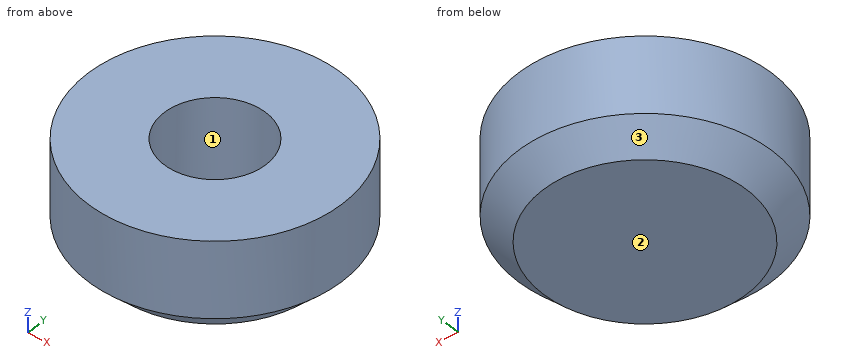
```python
from build123d import *

# Parameters (mm, degrees)
SKETCH_1_R      = 15
EXTRUDE_1_DEPTH = 2
SKETCH_2_R      = 15
SKETCH_2_R_2    = 6
EXTRUDE_2_DEPTH = 10
CHAMFER_1_SIZE  = 3


with BuildPart() as part:
    # 草图1 → 凸台-拉伸1 (new body)
    with BuildSketch(Plane.XY):
        Circle(SKETCH_1_R)
    extrude(amount=EXTRUDE_1_DEPTH)

    # 草图2 → 凸台-拉伸2 (add)
    with BuildSketch(Plane.XY.offset(2)):
        Circle(SKETCH_2_R)
        Circle(SKETCH_2_R_2, mode=Mode.SUBTRACT)
    extrude(amount=EXTRUDE_2_DEPTH)

    # 倒角1
    chamfer_1_edges = [part.edges().sort_by_distance(p)[0] for p in [
        (-15, 0, 0),
    ]]
    chamfer(chamfer_1_edges, length=CHAMFER_1_SIZE)


solid = part.part
```
The listing builds one solid part. Answer for the finished solid, in the listing's coordinates (mm). Face numbers are marked on the shaded views. Round coordinates to 2 decimals unless told otherwise and drop trailing zeros. Write each loop counter-clockwise with the first axis right and the second up, starting at its lowest first coordinate (ties: lowest second). Pieces come first, ordered by that corner, then holes. Notation, with made-up numbers: (7.25, -17.5) -> (46.25, -17.5) arc R22 cw to (46.25, 2.5) -> close; hole circle Ø3 at (45, 33). An arc over 180 degrees is marked (long way). Answer as a JSON object with one key per item and string values. Group by question number.
Q1. Section C-C (z = 8.75) is taken. Write down the section's boundary in (x, y).
Q2. Straight lines are drawn through the part: line 1 along Y through (x, z) = (0, 6); line 2 along Y through (x, z) = (-4.75, 10.5); line 3 along Z through (x, y) = (2.25, 2.25). For each, find the intervals that lie inside material, in ascending order.
Q3. Determine the mould class of the marked faces 1, 2 and 3 for opening direction X: pulls with the +X half, pulls with the -X half, needs draft (parallel to the pull), parting line crosses it, or undercut.
Q4. Section D-D (z = 1) is taken. Write down the section's boundary in (x, y), plus the area to 3 significant figures.
Q5. Each of these flat-tipped pins is pushed along its axis until it touches: pin 1 Ø1.5 at (y, z) = (-12, 4) entering from -X; pin 2 Ø3 at (y, z) = (4, 5.5) entering from +X; pin 3 Ø2 at (y, z) = (8, 5) entering from -X; pin 4 Ø6 at (x, y) = (-0.5, -3) entering from +Z. Where does it stop, or does it pass through?
Q6. Section A-A (x = 0) is taken. Write down the section's boundary in (y, z).
Check values:
{
 "1": {"outline": "circle Ø30 at (0, 0); hole circle Ø12 at (0, 0)"},
 "2": {"line 1": "-15 to -6, 6 to 15", "line 2": "-14.23 to -3.67, 3.67 to 14.23", "line 3": "0 to 2"},
 "3": {"face 1": "undercut", "face 2": "needs draft", "face 3": "parting line crosses it"},
 "4": {"outline": "circle Ø26 at (0, 0)", "area": "531 mm^2"},
 "5": {"pin 1": "x = -9.92", "pin 2": "x = 14.79", "pin 3": "x = -13.27", "pin 4": "z = 12"},
 "6": {"outline": "(-15, 3) -> (-12, 0) -> (12, 0) -> (15, 3) -> (15, 12) -> (6, 12) -> (6, 2) -> (-6, 2) -> (-6, 12) -> (-15, 12) -> close"}
}
